Read the model definition and answer for the solid it produces. Units are mm, in the model's axes. Face numbers are marked on the shaded views. A direction names the side the tool comes from. Give positions to 0.01 mm unless a question says otherwise; leave off trailing zeros. Order: outer loops, then holes, each group sorted by start corner. A loop starts at its lowest first (then second) coordinate and runs counter-clockwise, first axis right, second up. Notation, with made-up numbers: (-4.75, 40) - (26.25, 40) arc R31 ccw to (26.25, 77) - close; hole circle Ø1 at (27, -21.75). An arc over 180 degrees is marked (long way). Answer as CSV lines item,"result". Start each with the question number.
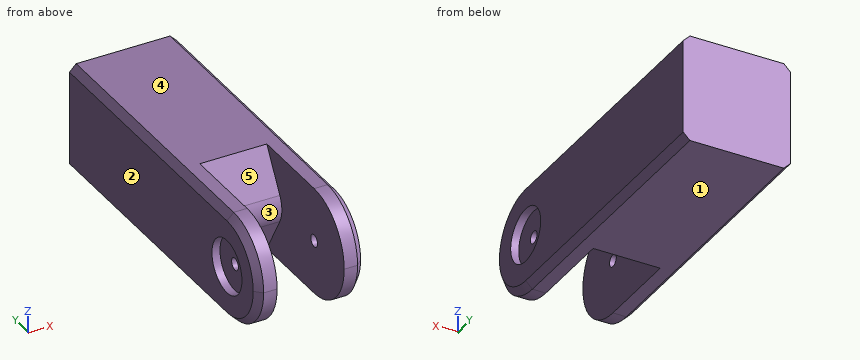
from build123d import *

# Parameters (mm, degrees)
F0_W      = 250
F0_H      = 80
F1_DEPTH  = 40
F2_R      = 39.99999
F4_DEPTH  = 25
F5_R      = 20
F6_SIZE   = 5
F7_R      = 4.5
F8_DEPTH  = 80.001
F9_R      = 20
F10_DEPTH = 6


# Not quite as in the source:
# - a fillet or chamfer is up to 0.001 mm smaller than in the source, because OpenCascade refuses the exact size
# - a pattern or mirror of a feature is missing from the dataset's text; its kind, count and spacing are read off the source's solid


with BuildPart() as f1:
    # F0 (on Right) → F1 (new body, symmetric)
    with BuildSketch(Plane.YZ):
        Rectangle(F0_W, F0_H)
    extrude(amount=F1_DEPTH, both=True)

    # F2 (radius 40 in the source; OpenCascade refuses exactly that, so slightly less here)
    f2_edges = [f1.edges().sort_by_distance(p)[0] for p in [
        (0, -125, 40),
        (0, -125, -40),
    ]]
    fillet(f2_edges, radius=F2_R)

    # F3 (on Right) → F4 (cut, symmetric)
    with BuildSketch(Plane.YZ):
        Polygon((-21.9059892324, -40), (-45, 0), (-21.9059892324, 40), (-155.967399478, 40), (-155.967399478, -40), align=None)
    extrude(amount=F4_DEPTH, both=True, mode=Mode.SUBTRACT)

    # F5
    f5_edges = [f1.edges().sort_by_distance(p)[0] for p in [
        (0, -45, 0),
    ]]
    fillet(f5_edges, radius=F5_R)

    # F6
    f6_edges = [f1.edges().sort_by_distance(p)[0] for p in [
        (40, 19.999995, 40),
        (-40, 19.999995, 40),
        (40, -113.284274, 28.284274),
        (40, 19.999995, -40),
        (-40, 19.999995, -40),
        (40, -125, 0),
        (40, -113.284274, -28.284274),
        (-40, -113.284274, 28.284274),
        (-40, -125, 0),
        (-40, -113.284274, -28.284274),
    ]]
    chamfer(f6_edges, length=F6_SIZE)

    # F7 (on face) → F8 (cut, through all)
    with BuildSketch(Plane.YZ.offset(40)):
        with Locations((-85, 0)):
            Circle(F7_R)
    extrude(amount=-F8_DEPTH, mode=Mode.SUBTRACT)

    # F9 (on face) → F10 (cut)
    with BuildSketch(Plane.YZ.offset(40)):
        with Locations((-85, 0)):
            Circle(F9_R)
    f10 = extrude(amount=-F10_DEPTH, mode=Mode.SUBTRACT)

    # F10_copies: F10 across plane
    add(f10.mirror(Plane(origin=(0, 0, 0), x_dir=(0, 0, -1), z_dir=(-1, 0, 0))), mode=Mode.SUBTRACT)


solid = f1.part
(1) Flat-ended cylindrical pins translate along their axes: pin 1 Ø11.5 at (y, z) = (-85, 0) entering from -X; pin 2 Ø4 at (x, z) = (-21.5, 29.5) entering from -Y; pin 3 Ø3 at (x, z) = (-11.5, -13.5) entering from -Y. Find the tip coordinate at first contact, or state that the pin passes through.
(2) Which of the six approach directions +Z, -Z, +X, -X, +Y, -Y give full straight-line access (tool end or side, diameter ignored) to the marked faces 4 and 5?
(3) Determine the mould class of the marked faces 1, 2 and 3 for opening direction X: released by +X, released by -X, zero draft, split by the parting line, or undercut.
(4) Section D-D, the plane x = -21.5 is taken. Write down the section's boundary in (y, z).
(5) Section C-C, the plane y = -28.5 is taken. Write down the section's boundary in (x, z), and give its area (3 significant figures).
(6) Straight lines are drawn through the part: line 1 (X direction, y = -52.5, z = -19.5); line 2 (X direction, y = -85, z = -15.5); line 3 (Z direction, x = -38, y = -85). For each, find the intervals that lie inside material, in ascending order. Write a range as [from, to].
(7) Section A-A, the plane y = -60.5 is taken. Write down the section's boundary in (x, z).
Checks:
1,pin 1,"stops at x = -34"
1,pin 2,"stops at y = -29.12"
1,pin 3,"stops at y = -38.07"
2,face 4,"+Z, +X, -X, +Y, -Y"
2,face 5,"+Z, -Y"
3,face 1,"zero draft"
3,face 2,"released by -X"
3,face 3,"undercut"
4,outline,"(-39.23, -10) - (-21.91, -40) - (125, -40) - (125, 40) - (-21.91, 40) - (-39.23, 10) arc R20 ccw to start"
5,outline,"(-40, -35) - (-35, -40) - (-25, -40) - (-25, -28.58) - (25, -28.58) - (25, -40) - (35, -40) - (40, -35) - (40, 35) - (35, 40) - (25, 40) - (25, 28.58) - (-25, 28.58) - (-25, 40) - (-35, 40) - (-40, 35) - close"
5,area,"5,210 mm²"
6,line 1,"x = [-40, -25], [25, 40]"
6,line 2,"x = [-34, -25], [25, 34]"
6,line 3,"z = [-37, -20], [20, 37]"
7,outline,"(-40, -35) - (-35, -40) - (-25, -40) - (-25, 40) - (-35, 40) - (-40, 35) - close; (25, -40) - (35, -40) - (40, -35) - (40, 35) - (35, 40) - (25, 40) - close"
